Input: part model. Units: mm. Frame: model coordinates. Coordinates: 2 decimals unless noted, no trailing zeros. Write each loop counter-clockwise with the first axis right and the second up, starting at its lowest first coordinate (ties: lowest second). Pieces come first, ordered by that corner, then holes.
from build123d import *

# Parameters (mm, degrees)
SKETCH_1_R          = 60
SKETCH_1_R_2        = 1.5
EXTRUDE_1_DEPTH     = 2
SKETCH_3_R          = 11.5
CUT_EXTRUDE_3_DEPTH = 2
SKETCH_4_R          = 1.5
CUT_EXTRUDE_4_DEPTH = 2
SKETCH_5_R          = 3
CUT_EXTRUDE_5_DEPTH = 10
SKETCH_6_R          = 2
CUT_EXTRUDE_6_DEPTH = 10
SKETCH_7_R          = 3
CUT_EXTRUDE_7_DEPTH = 10
SKETCH_8_R          = 3
CUT_EXTRUDE_8_DEPTH = 10
SKETCH_9_R          = 1.5
CUT_EXTRUDE_9_DEPTH = 10


with BuildPart() as part:
    # 草图1 → 凸台-拉伸1 (new body)
    with BuildSketch(Plane(origin=(0, 0, 0), x_dir=(1, 0, 0), z_dir=(0, 1, 0))):
        with Locations(Location((0, 0, 0), (0, 0, 270))):
            Circle(SKETCH_1_R)
        with Locations(Location((0, 31, 0), (0, 0, 270))):
            Circle(SKETCH_1_R_2, mode=Mode.SUBTRACT)
        with Locations(Location((26.846787517, -15.5, 0), (0, 0, 270))):
            Circle(SKETCH_1_R_2, mode=Mode.SUBTRACT)
        with Locations(Location((-26.846787517, -15.5, 0), (0, 0, 270))):
            Circle(SKETCH_1_R_2, mode=Mode.SUBTRACT)
    extrude(amount=EXTRUDE_1_DEPTH)

    # 草图3 → 切除-拉伸3 (cut)
    with BuildSketch(Plane(origin=(0, 2, 0), x_dir=(1, 0, 0), z_dir=(0, 1, 0))):
        with Locations(Location((0, 0, 0), (0, 0, 270))):
            Circle(SKETCH_3_R)
    extrude(amount=-CUT_EXTRUDE_3_DEPTH, mode=Mode.SUBTRACT)

    # 草图4 → 切除-拉伸4 (cut)
    with BuildSketch(Plane(origin=(0, 2, 0), x_dir=(1, 0, 0), z_dir=(0, 1, 0))):
        with Locations(Location((-15.5, 15.5, 0), (0, 0, 270))):
            Circle(SKETCH_4_R)
        with Locations(Location((15.5, 15.5, 0), (0, 0, 270))):
            Circle(SKETCH_4_R)
        with Locations(Location((15.5, -15.5, 0), (0, 0, 270))):
            Circle(SKETCH_4_R)
        with Locations(Location((-15.5, -15.5, 0), (0, 0, 270))):
            Circle(SKETCH_4_R)
    extrude(amount=-CUT_EXTRUDE_4_DEPTH, mode=Mode.SUBTRACT)

    # 草图5 → 切除-拉伸5 (cut)
    with BuildSketch(Plane.XZ):
        with Locations(Location((10, -14.64, 0), (0, 0, 270))):
            Circle(SKETCH_5_R)
        with Locations(Location((-10, -14.64, 0), (0, 0, 270))):
            Circle(SKETCH_5_R)
    extrude(amount=-CUT_EXTRUDE_5_DEPTH, mode=Mode.SUBTRACT)

    # 草图6 → 切除-拉伸6 (cut)
    with BuildSketch(Plane.XZ):
        with Locations(Location((0, 55, 0), (0, 0, 270))):
            Circle(SKETCH_6_R)
        with Locations(Location((55, 0, 0), (0, 0, 270))):
            Circle(SKETCH_6_R)
        with Locations(Location((0, -55, 0), (0, 0, 270))):
            Circle(SKETCH_6_R)
        with Locations(Location((-55, 0, 0), (0, 0, 270))):
            Circle(SKETCH_6_R)
    extrude(amount=-CUT_EXTRUDE_6_DEPTH, mode=Mode.SUBTRACT)

    # 草图7 → 切除-拉伸7 (cut)
    with BuildSketch(Plane.XZ):
        with Locations(Location((10, -35, 0), (0, 0, 270))):
            Circle(SKETCH_7_R)
        with Locations(Location((-10, -35, 0), (0, 0, 270))):
            Circle(SKETCH_7_R)
    extrude(amount=-CUT_EXTRUDE_7_DEPTH, mode=Mode.SUBTRACT)

    # 草图8 → 切除-拉伸8 (cut)
    with BuildSketch(Plane.XZ):
        with Locations(Location((31.6, -35, 0), (0, 0, 270))):
            Circle(SKETCH_8_R)
        with Locations(Location((-31.6, -35, 0), (0, 0, 270))):
            Circle(SKETCH_8_R)
    extrude(amount=-CUT_EXTRUDE_8_DEPTH, mode=Mode.SUBTRACT)

    # 草图9 → 切除-拉伸9 (cut)
    with BuildSketch(Plane.XZ):
        with Locations(Location((-31.6, -14.64, 0), (0, 0, 270))):
            Circle(SKETCH_9_R)
        with Locations(Location((31.6, -14.64, 0), (0, 0, 270))):
            Circle(SKETCH_9_R)
    extrude(amount=-CUT_EXTRUDE_9_DEPTH, mode=Mode.SUBTRACT)


solid = part.part
Item 1: Section query D-D, the plane x = 15.5. Return loops of the section in (y, z).
Item 2: Section query A-A, the plane z = 0. Return loops of the section in (x, y).
Item 3: Pin query (flat end, axial travel): pin 1 Ø1 at (x, y) = (-6.5, 2) entering from +Z. Return the tip coordinate at first contact, or that it passes through.
Item 4: Pull-direction query (Z, two-part tool) for faces 1 (the face through (2.64, 0.99, -59.94)), 2 (the face through (10, 1, -32)), 3 (the face through (1, 0, 12)); classes: released by +Z, released by -Z, zero draft, split by the parting line, or undercut.
Item 5: Section query C-C, the plane z = 15.5. Return loops of the section in (x, y).
Item 6: Material intervals for line 1 (Z direction, x = -49, y = 0.35); line 2 (Z direction, x = -25.5, y = 0.3); line 3 (X direction, y = 1.3, z = -12), sorted ascending.
Item 7: Section query B-B, the plane x = 55. Return loops of the section in (y, z), then the cut area to 3 significant figures.
The answers:
1. outline: (0, -57.96) - (2, -57.96) - (2, -17) - (0, -17) - close; (0, -14) - (2, -14) - (2, 14) - (0, 14) - close; (0, 17) - (2, 17) - (2, 57.96) - (0, 57.96) - close
2. outline: (-60, 0) - (-57, 0) - (-57, 2) - (-60, 2) - close; (-53, 0) - (-11.5, 0) - (-11.5, 2) - (-53, 2) - close; (11.5, 0) - (53, 0) - (53, 2) - (11.5, 2) - close; (57, 0) - (60, 0) - (60, 2) - (57, 2) - close
3. pin 1: stops at z = 59.7
4. face 1: split by the parting line
4. face 2: undercut
4. face 3: zero draft
5. outline: (-57.96, 0) - (-28.35, 0) - (-28.35, 2) - (-57.96, 2) - close; (-25.35, 0) - (-17, 0) - (-17, 2) - (-25.35, 2) - close; (-14, 0) - (14, 0) - (14, 2) - (-14, 2) - close; (17, 0) - (25.35, 0) - (25.35, 2) - (17, 2) - close; (28.35, 0) - (57.96, 0) - (57.96, 2) - (28.35, 2) - close
6. line 1: z = -34.63 to 34.63
6. line 2: z = -54.31 to 14.84, 16.16 to 54.31
6. line 3: x = -58.79 to -11.42, -8.58 to 8.58, 11.42 to 58.79
7. outline: (0, -23.98) - (2, -23.98) - (2, -2) - (0, -2) - close; (0, 2) - (2, 2) - (2, 23.98) - (0, 23.98) - close
7. area: 87.9 mm2
